Input: part model. Units: mm. Frame: model coordinates. Face numbers are marked on the shaded views. A direction names the side the tool comes from. Round coordinates to 2 decimals unless told otherwise and drop trailing zeros. Order: outer loops, then holes, each group sorted by start corner. A loop starts at its lowest first (then second) coordinate and runs counter-clockwise, first axis right, second up. Notation, with made-up numbers: (66.5, 61) -> (125.5, 61) arc R26 cw to (125.5, 84) -> close; hole circle Ø3 at (50, 58). An arc over 180 degrees is marked (long way). Use a Markdown table: item, result.
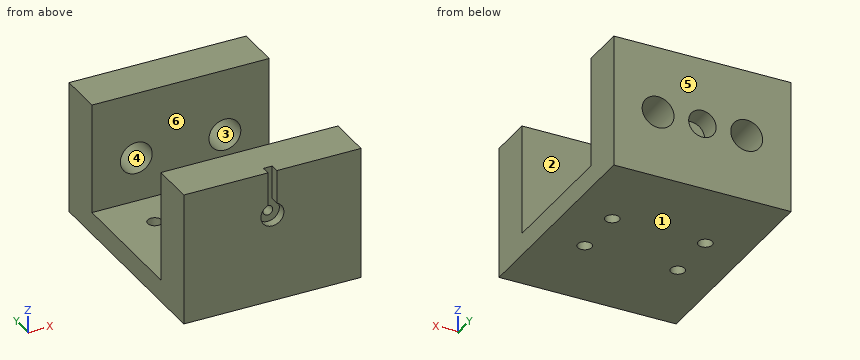
from build123d import *

# Parameters (mm, degrees)
F1_DEPTH = 20
F2_R     = 1.6
F3_DEPTH = 25
F4_R     = 1.1
F5_DEPTH = 25
F6_DEPTH = 2
F7_R     = 3.6
F8_DEPTH = 25
F7_R_2   = 3.1
F9_DEPTH = 5


with BuildPart() as f1:
    # F0 (on Right) → F1 (new body, symmetric)
    with BuildSketch(Plane.YZ):
        Polygon((-25, -15), (25, -15), (25, 15), (15, 15), (15, -10), (-15, -10), (-15, 15), (-25, 15), align=None)
    extrude(amount=F1_DEPTH, both=True)

    # F2 (on face) → F3 (cut)
    with BuildSketch(Plane(origin=(0, 0, -15), x_dir=(1, 0, 0), z_dir=(0, 0, -1))):
        with Locations((10.5, 6)):
            Circle(F2_R)
        with Locations((10.5, -6)):
            Circle(F2_R)
        with Locations((-10.5, 6)):
            Circle(F2_R)
        with Locations((-10.5, -6)):
            Circle(F2_R)
    extrude(amount=-F3_DEPTH, mode=Mode.SUBTRACT)

    # F4 (on face) → F5 (cut)
    with BuildSketch(Plane.XZ.offset(25)):
        with Locations((0, 5)):
            Circle(F4_R)
    extrude(amount=-F5_DEPTH, mode=Mode.SUBTRACT)

    # F4 (on face) → F6 (cut)
    with BuildSketch(Plane.XZ.offset(25)):
        with BuildLine():
            Line((-1, 15), (-1, 7.4))
            ThreePointArc((-1, 7.4), (0, 2.4), (1, 7.4))
            Line((1, 7.4), (1, 15))
            Line((1, 15), (-1, 15))
        make_face()
        with Locations((0, 5)):
            Circle(F4_R, mode=Mode.SUBTRACT)
    extrude(amount=-F6_DEPTH, mode=Mode.SUBTRACT)

    # F7 (on face) → F8 (cut)
    with BuildSketch(Plane(origin=(0, 25, 0), x_dir=(-1, 0, 0), z_dir=(0, 1, 0))):
        with Locations((-10, 0)):
            Circle(F7_R)
        with Locations((10, 0)):
            Circle(F7_R)
    extrude(amount=-F8_DEPTH, mode=Mode.SUBTRACT)

    # F7 (on face) → F9 (cut)
    with BuildSketch(Plane(origin=(0, 25, 0), x_dir=(-1, 0, 0), z_dir=(0, 1, 0))):
        Circle(F7_R_2)
    extrude(amount=-F9_DEPTH, mode=Mode.SUBTRACT)


solid = f1.part
1) Cut plane A-A on y = -6. Return loops of the section in (x, z).
Answer key:
| item | result |
|---|---|
| outline | (-20, -15) -> (-12.1, -15) -> (-12.1, -10) -> (-20, -10) -> close; (-8.9, -15) -> (8.9, -15) -> (8.9, -10) -> (-8.9, -10) -> close; (12.1, -15) -> (20, -15) -> (20, -10) -> (12.1, -10) -> close |
2) Draft query along Y for the marked faces 4, 5 and 6. Return one class per face: released by +Y, released by -Y, zero draft, split by the parting line, or undercut.
Answer key:
| item | result |
|---|---|
| face 4 | zero draft |
| face 5 | released by +Y |
| face 6 | undercut |
3) Cut plane C-C on z = 5. Return loops of the section in (x, y).
Answer key:
| item | result |
|---|---|
| outline | (-20, -25) -> (-2.6, -25) -> (-2.6, -23) -> (-1.1, -23) -> (-1.1, -15) -> (-20, -15) -> close; (-20, 15) -> (20, 15) -> (20, 25) -> (-20, 25) -> close; (1.1, -23) -> (2.6, -23) -> (2.6, -25) -> (20, -25) -> (20, -15) -> (1.1, -15) -> close |
4) Set-up query: the marked faces 1, 2 and 3. Return all of +Z, -Z, +X, -X, +Y, -Y with unobstructed straight access to the full face (end or side cutting, diameter ignored); none if empty.
Answer key:
| item | result |
|---|---|
| face 1 | -Z, +X, -X, +Y, -Y |
| face 2 | +Z, +X, -X |
| face 3 | +Y |
5) Cut plane D-D on x = 10.5. Return loops of the section in (y, z), and give its area (3 significant figures).
Answer key:
| item | result |
|---|---|
| outline | (-25, -15) -> (-7.6, -15) -> (-7.6, -10) -> (-15, -10) -> (-15, 15) -> (-25, 15) -> close; (-4.4, -15) -> (4.4, -15) -> (4.4, -10) -> (-4.4, -10) -> close; (7.6, -15) -> (25, -15) -> (25, -3.57) -> (15, -3.57) -> (15, -10) -> (7.6, -10) -> close; (15, 3.57) -> (25, 3.57) -> (25, 15) -> (15, 15) -> close |
| area | 647 mm^2 |
6) Contact query for flat-ended pins moving along their axis: P1, Ø6, axis at x = 3.5, y = 2.5, coming from the +Z side; P2, Ø1.3, axis at x = 0, z = 5, coming from the -Y side; P3, Ø1.9, axis at x = -10.5, y = -6, coming from the -Z side; P4, Ø3, axis at x = 0, z = 5, coming from the -Y side. Output: stop coordinate, or through.
Answer key:
| item | result |
|---|---|
| P1 | stops at z = -10 |
| P2 | stops at y = 15 |
| P3 | passes through |
| P4 | stops at y = -23 |
7) Cut plane B-B on z = -5.75. Return loops of the section in (x, y), and give its area (3 significant figures).
Answer key:
| item | result |
|---|---|
| outline | (-20, -25) -> (20, -25) -> (20, -15) -> (-20, -15) -> close; (-20, 15) -> (20, 15) -> (20, 25) -> (-20, 25) -> close |
| area | 800 mm^2 |
8) Ray query, probe 1 along X at (y, z) = (6, -13.35); probe 2 along Y at (x, z) = (-15.5, 0.5); probe 3 along Y at (x, z) = (10.5, -12.4). Return the intervals inside material, ascending.
Answer key:
| item | result |
|---|---|
| probe 1 | x = -20 to -12.1, -8.9 to 8.9, 12.1 to 20 |
| probe 2 | y = -25 to -15, 15 to 25 |
| probe 3 | y = -25 to -7.6, -4.4 to 4.4, 7.6 to 25 |
